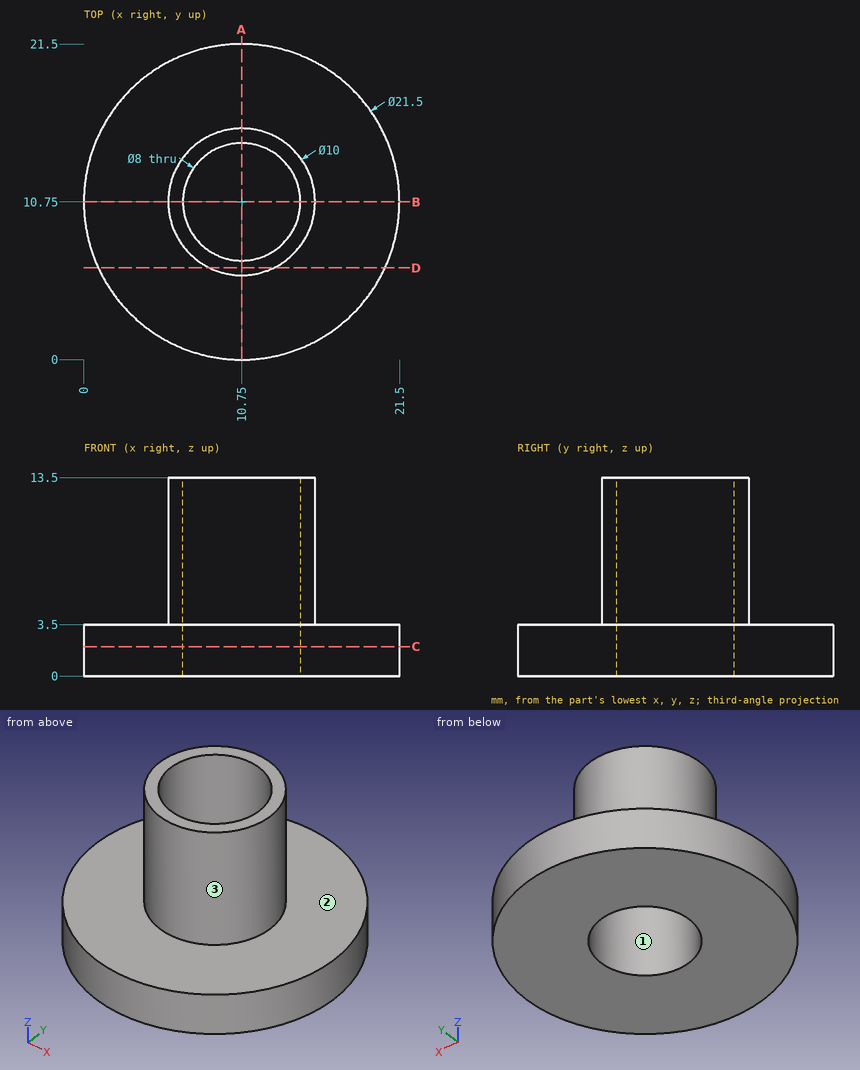
Geometry check sheet. Reference: drawing and pictorial views, mm from the part's lowest x, y, z. Give positions to 0.01 mm unless a question says otherwise; leave off trailing zeros. Loops run counter-clockwise (first coordinate to the right, second up) from the corner with the lowest first, then second, coordinate; pieces in that order, holes last. Notation, with made-up numbers: M -26.75,51.25 L -17.75,51.25 A14 ccw -17.75,67.25 Z; hole C 69,-38 d6. An arc over 180 degrees is marked long. Use a Markdown table: item, result. Add a question column.
Q1. Sectioned sample at A-A, the plane x = 10.75. Record the cut outline in (y, z), then the cut area to 4 significant figures.
Q2. Go/stop test with flat-tipped pins: pin 1 (8 mm diameter, centred on y = 19, z = 9, fed in from -X); pin 2 (2 mm diameter, centred on y = 14.5, z = 3.5, fed in from -X); pin 3 (5 mm diameter, centred on x = 2.5, y = 6, fed in from +Z). Record where each tip stops, or that it passes through.
Q3. Sectioned sample at D-D, the plane y = 6.25. Record the cut outline in (x, z), then the cut area to 3 significant figures.
Q4. Sectioned sample at C-C, the plane z = 2. Record the cut outline in (x, y), then the cut area to 3 significant figures.
Q5. Mould release check, pull along Y, two halves, no side actions. Record for the marked faces 1, 2 and 3: pulls with the +Y half, pulls with the -Y half, needs draft (parallel to the pull), parting line crosses it, or undercut.
Q6. Scan lines: line 1 along Y through (x, z) = (10.75, 6.25); line 2 along Y through (x, z) = (10.75, 2.75); line 3 along Z through (x, y) = (5, 12.5). Record each from-to range of solid material in increasing order. Write a range as [from, to].
Verdict:
| question | item | result |
|---|---|---|
| 1 | outline | M 0,0 L 6.75,0 L 6.75,13.5 L 5.75,13.5 L 5.75,3.5 L 0,3.5 Z; M 14.75,0 L 21.5,0 L 21.5,3.5 L 15.75,3.5 L 15.75,13.5 L 14.75,13.5 Z |
| 1 | area | 67.25 mm^2 |
| 2 | pin 1 | x = 8.12 |
| 2 | pin 2 | x = 0.36 |
| 2 | pin 3 | z = 3.5 |
| 3 | outline | M 0.99,0 L 20.51,0 L 20.51,3.5 L 12.93,3.5 L 12.93,13.5 L 8.57,13.5 L 8.57,3.5 L 0.99,3.5 Z |
| 3 | area | 112 mm^2 |
| 4 | outline | C 10.75,10.75 d21.5; hole C 10.75,10.75 d8 |
| 4 | area | 313 mm^2 |
| 5 | face 1 | undercut |
| 5 | face 2 | needs draft |
| 5 | face 3 | parting line crosses it |
| 6 | line 1 | [5.75, 6.75], [14.75, 15.75] |
| 6 | line 2 | [0, 6.75], [14.75, 21.5] |
| 6 | line 3 | [0, 3.5] |
